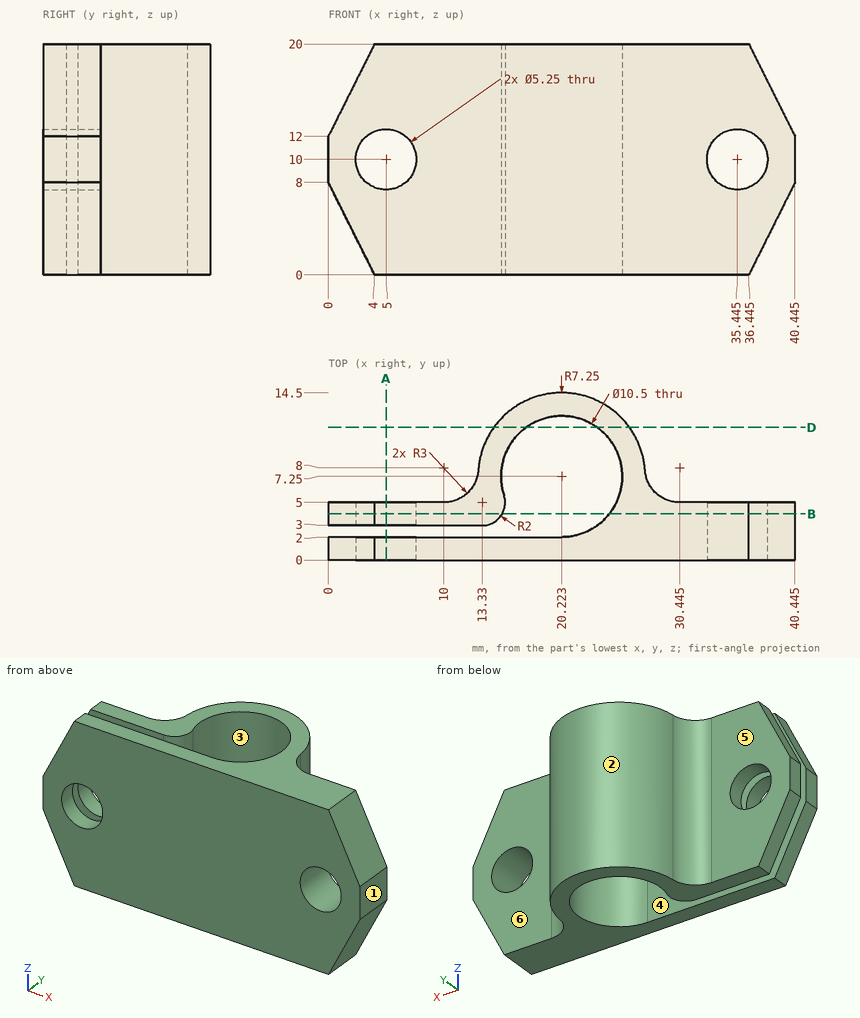
The figure shows three views and two pictorial views of one solid part (mm, origin at its lowest corner). Answer the questions. A direction names the side the tool comes from. Give positions to 0.01 mm unless a question says otherwise; leave off trailing zeros. Loops run counter-clockwise (first coordinate to the right, second up) from the corner with the lowest first, then second, coordinate; pieces in that order, holes last. Notation, with made-up numbers: (-34.5, -33.5) - (14.5, -33.5) arc R20 cw to (14.5, -25.5) - close; hole circle Ø8 at (1.25, 56.25). An arc over 180 degrees is marked (long way). Answer in a Markdown table with one row per item.
(1) Flat-ended cylindrical pins translate along their axes: pin 1 Ø1 at (x, z) = (11, 2.5) entering from +Y; pin 2 Ø8 at (x, z) = (4, 11) entering from +Y; pin 3 Ø4 at (x, z) = (24.5, 12) entering from +Y; pin 4 Ø4 at (x, z) = (35.45, 10) entering from -Y. Find the tip coordinate at first contact, or state that the pin passes through.
Results list:
| item | result |
|---|---|
| pin 1 | stops at y = 5.4 |
| pin 2 | stops at y = 5 |
| pin 3 | stops at y = 14.13 |
| pin 4 | passes through |
(2) Section A-A (x = 5) is taken. Give the vertices of the cut face in (y, z) (1 decimal).
Results list:
| item | result |
|---|---|
| outline | (0, 0) - (2, 0) - (2, 7.4) - (0, 7.4) - close; (0, 12.6) - (2, 12.6) - (2, 20) - (0, 20) - close; (3, 0) - (5, 0) - (5, 7.4) - (3, 7.4) - close; (3, 12.6) - (5, 12.6) - (5, 20) - (3, 20) - close |
(3) A tool of negligible diameter and unlimited length cuts with its end or side. For the marked faces 4, 5 and 6, from which of +Z, -Z, +X, -X, +Y, -Y can it reach the whole face along a straight path? Write none if from no direction.
Results list:
| item | result |
|---|---|
| face 4 | +Z, -Z, -X |
| face 5 | +Z, -Z, -X, +Y |
| face 6 | +Z, -Z, +X, +Y |
(4) Section D-D (y = 11.5) is taken. Give the vertices of the cut face in (x, z) (1 decimal).
Results list:
| item | result |
|---|---|
| outline | (14.3, 0) - (17.1, 0) - (17.1, 20) - (14.3, 20) - close; (23.3, 0) - (26.1, 0) - (26.1, 20) - (23.3, 20) - close |
(5) For a pull along X with two mould halves and no side action, classify the marked faces 1, 2 and 3 as pulls with the +X half, pulls with the -X half, needs draft (parallel to the pull), parting line crosses it, or undercut.
Results list:
| item | result |
|---|---|
| face 1 | pulls with the +X half |
| face 2 | parting line crosses it |
| face 3 | undercut |
(6) Section B-B (y = 4) is taken. State how many separate pieces and enclosed holes the cut face has, and give its area (3 significant figures).
Results list:
| item | result |
|---|---|
| separate pieces | 2 |
| enclosed holes | 2 |
| area | 516 mm² |
(7) Consider L1, parallel to Y at x = 7, z = 13.5; L2, parallel to Y at x = 25, z = 18.75 (1 decimal); L3, parallel to X at y = 3.75, z = 18.25 (1 decimal). Determine where each line is inside the solid, lowest interval first. Write a range as [from, to].
Results list:
| item | result |
|---|---|
| L1 | y = [0, 2], [3, 5] |
| L2 | y = [0, 5.1], [9.4, 12.7] |
| L3 | x = [3.1, 14.9], [24.1, 37.3] |
